Geometry check sheet. Reference: the model listing, model coordinates, mm. A direction names the side the tool comes from. Give positions to 0.01 mm unless a question says otherwise; leave off trailing zeros. Loops run counter-clockwise (first coordinate to the right, second up) from the corner with the lowest first, then second, coordinate; pieces in that order, holes last. Notation, with made-up numbers: (77.25, 73) -> (97.25, 73) arc R22 ccw to (97.25, 95) -> close; hole circle Ø10 at (26.5, -30.75). An arc over 180 degrees is marked (long way). One line per item, written item: value. Start each with the question number.
(1) Sectioned sample at D-D, the plane x = 0.75. Record the cut outline in (y, z), then the cut area to 3 significant figures.
(2) Draft check along Z on faces 1 (the face through (4.4, 25, -317.2)), 2 (the face through (1.126, 24.715, -328.563)), 3 (the face through (1.79, 16.52, -315.82)). Enter one of: pulls with the +Z half, pulls with the -Z half, needs draft (parallel to the pull), parting line crosses it, or undercut.
(3) Scan lines: line 1 along Z through (x, y) = (-6.5, 23.75); line 2 along Y through (x, z) = (-3.5, -317); line 3 along Z through (x, y) = (0.75, 24). Record each from-to range of solid material in increasing order. Write a range as from..to.
(4) Gauge pin test, flat end, axial feed: pin 1 Ø3 at (x, z) = (-1.5, -315.5) entering from +Y. Record the tip position at first contact, or that the pin passes through.
(5) Sectioned sample at A-A, the plane y = 16.75. Record the cut outline in (x, z), then the cut area to 3 significant figures.
(6) Tool access check on faces 4 (the face through (9.715, 24.699, -314.073)), 5 (the face through (-4, 18, -314)). Record the directions out of +Z, -Z, +X, -X, +Y, -Y that give a thin tool (end or side, any length) a straight path to the whole face; none if there is none.
(7) Sectioned sample at B-B, the plane x = -4.5. Record the cut outline in (y, z).
from build123d import *

# Parameters (mm, degrees)
SKETCH2_W          = 20
SKETCH2_H          = 30
EXTRUDE1_DEPTH     = 10
CUT_EXTRUDE1_DEPTH = 7
SKETCH4_R          = 2.65
CUT_EXTRUDE2_DEPTH = 17
SKETCH7_W          = 2
SKETCH7_H          = 10
EXTRUDE2_DEPTH     = 30
FILLET1_R          = 1


with BuildPart() as part:
    # Sketch2 → Extrude1 (new body)
    with BuildSketch(Plane(origin=(0, 15, 0), x_dir=(1, 0, 0), z_dir=(0, 1, 0))):
        with Locations((0, 313.863465254)):
            Rectangle(SKETCH2_W, SKETCH2_H)
    extrude(amount=EXTRUDE1_DEPTH)

    # Sketch3 → Cut-Extrude1 (cut)
    with BuildSketch(Plane(origin=(0, 25, 0), x_dir=(1, 0, 0), z_dir=(0, 1, 0))):
        with BuildLine():
            Line((0, 319.063465254), (-7, 319.063465254))
            Line((-7, 319.063465254), (-7, 308.663465254))
            Line((-7, 308.663465254), (0, 308.663465254))
            ThreePointArc((0, 308.663465254), (5.2, 313.863465254), (0, 319.063465254))
        make_face()
    extrude(amount=-CUT_EXTRUDE1_DEPTH, mode=Mode.SUBTRACT)

    # Sketch4 → Cut-Extrude2 (cut)
    with BuildSketch(Plane(origin=(0, 18, 0), x_dir=(1, 0, 0), z_dir=(0, 1, 0))):
        with Locations(Location((0, 313.863465254, 0), (0, 0, 270))):
            Circle(SKETCH4_R)
    extrude(amount=-CUT_EXTRUDE2_DEPTH, mode=Mode.SUBTRACT)

    # Sketch7 → Extrude2 (cut)
    with BuildSketch(Plane.XY.offset(-298.863465254)):
        with Locations((-9, 20)):
            Rectangle(SKETCH7_W, SKETCH7_H)
    extrude(amount=-EXTRUDE2_DEPTH, mode=Mode.SUBTRACT)

    # Fillet1
    fillet1_edges = [part.edges().sort_by_distance(p)[0] for p in [
        (1, 25, -298.863465254),
        (-8, 25, -313.863465254),
        (10, 25, -313.863465254),
        (1, 25, -328.863465254),
    ]]
    fillet(fillet1_edges, radius=FILLET1_R - 0.0001)  # a hair under: the kernel refuses the full size


solid = part.part
Calculated:
1. outline: (15, -328.86) -> (24, -328.86) arc R1 ccw to (25, -327.86) -> (25, -319.01) -> (18, -319.01) -> (18, -316.41) -> (15, -316.41) -> close; (15, -311.32) -> (18, -311.32) -> (18, -308.72) -> (25, -308.72) -> (25, -299.86) arc R1 ccw to (24, -298.86) -> (15, -298.86) -> close
1. area: 212 mm2
2. face 1: needs draft
2. face 2: pulls with the -Z half
2. face 3: undercut
3. line 1: z = -328.86..-319.06, -308.66..-298.86
3. line 2: y = 15..18
3. line 3: z = -328.86..-319.01, -308.72..-298.86
4. pin 1: stops at y = 18
5. outline: (-8, -328.86) -> (10, -328.86) -> (10, -298.86) -> (-8, -298.86) -> close; hole circle Ø5.3 at (0, -313.86)
5. area: 518 mm2
6. face 4: +Z, -Z, +X, +Y
6. face 5: +Y
7. outline: (15, -328.86) -> (24, -328.86) arc R1 ccw to (25, -327.86) -> (25, -319.06) -> (18, -319.06) -> (18, -308.66) -> (25, -308.66) -> (25, -299.86) arc R1 ccw to (24, -298.86) -> (15, -298.86) -> close
